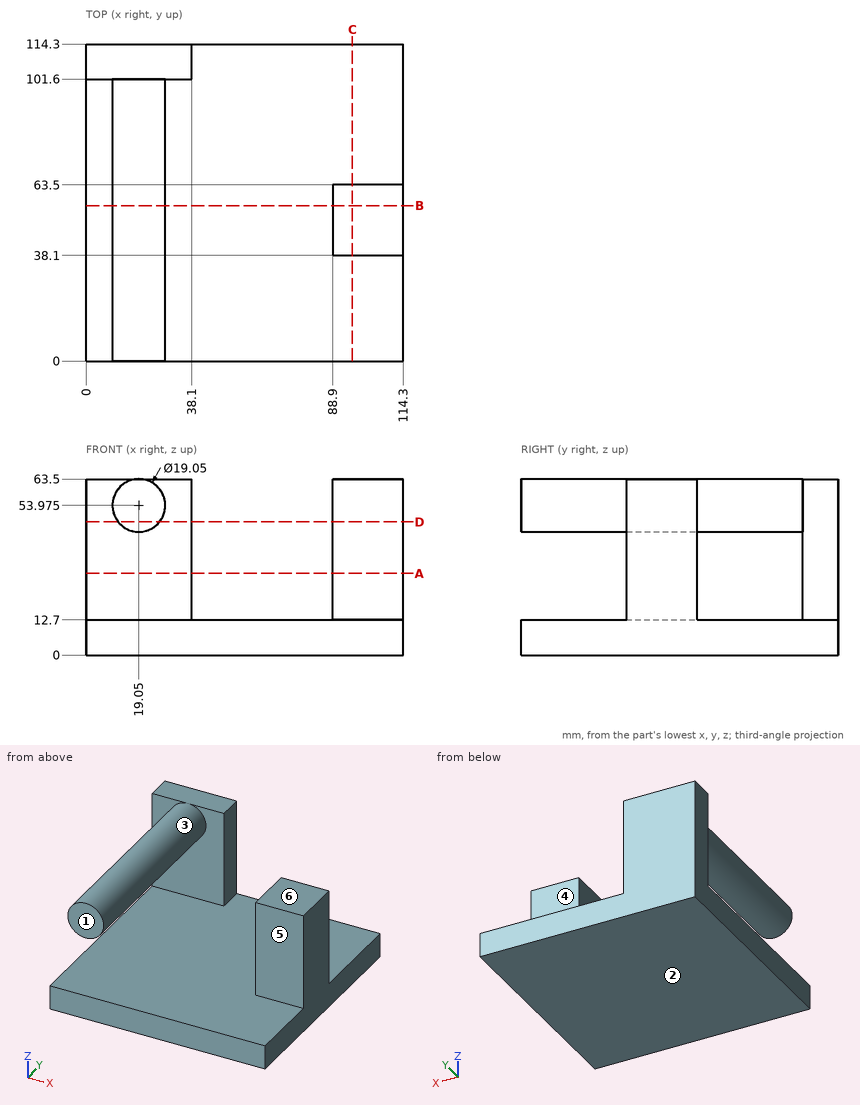
Design review of the part shown in the three views and the two pictorial views. Dimensions are in mm from the part's minimum x, y and z. A direction names the side the tool comes from. Round coordinates to 2 decimals unless told otherwise and drop trailing zeros. Order: outer loops, then holes, each group sorted by start corner. A loop starts at its lowest first (then second) coordinate and runs counter-clockwise, first axis right, second up.
Q1. We need section C-C, the plane x = 96. Give the boundary of the cut face in (y, z), plus the area to 3 significant figures.
Findings below:
outline: (0, 0) - (114.3, 0) - (114.3, 12.7) - (63.5, 12.7) - (63.5, 63.5) - (38.1, 63.5) - (38.1, 12.7) - (0, 12.7) - close
area: 2,740 mm2
Q2. Wall thickness on line 1 (Z direction, x = 62.5, y = 71); line 2 (Y direction, x = 37, z = 52.5); line 3 (X direction, y = 62, z = 27): over which ranges is each line inside the solid? List them lowest first.
Findings below:
line 1: z = 0 to 12.7
line 2: y = 101.6 to 114.3
line 3: x = 88.9 to 114.3
Q3. We need section A-A, the plane z = 29.5. Give the boundary of the cut face in (x, y), plus the area to 3 significant figures.
Findings below:
outline: (0, 101.6) - (38.1, 101.6) - (38.1, 114.3) - (0, 114.3) - close; (88.9, 38.1) - (114.3, 38.1) - (114.3, 63.5) - (88.9, 63.5) - close
area: 1,130 mm2
Q4. We need section D-D, the plane z = 48. Give the boundary of the cut face in (x, y).
Findings below:
outline: (0, 101.6) - (11.63, 101.6) - (11.63, 0) - (26.47, 0) - (26.47, 101.6) - (38.1, 101.6) - (38.1, 114.3) - (0, 114.3) - close; (88.9, 38.1) - (114.3, 38.1) - (114.3, 63.5) - (88.9, 63.5) - close
Q5. Mouldability with a two-part tool opening along Z and no side actions: class the marked faces 1, 2 and 3 as pulls with the +Z half, pulls with the -Z half, needs draft (parallel to the pull), parting line crosses it, or undercut.
Findings below:
face 1: needs draft
face 2: pulls with the -Z half
face 3: undercut
Q6. We need section B-B, the plane y = 56. Give the boundary of the cut face in (x, z) (3 decimals).
Findings below:
outline: (0, 0) - (114.3, 0) - (114.3, 63.5) - (88.9, 63.5) - (88.9, 12.7) - (0, 12.7) - close; circle Ø19.05 at (19.05, 53.975)
Q7. Insertion check: P1, Ø10, axis at y = 106.5, z = 27.5, coming from the +X side; P2, Ø12, axis at y = 67.5, z = 18.5, coming from the -X side; P3, Ø2, axis at x = 96.5, z = 30, coming from the -Y side; P4, Ø20.5, axis at x = 105, z = 27.5, coming from the +Y side. Each pin has a flat end and moves straight along its axis. Give the tip position at first contact, or say it passes through.
Findings below:
P1: stops at x = 38.1
P2: stops at x = 0
P3: stops at y = 38.1
P4: stops at y = 63.5
Q8. Machinability: for the marked faces 4, 5 and 6, which of the approach directions +Z, -Z, +X, -X, +Y, -Y give a long, thin tool a straight path to every point of the face, cutting with its end or side? Answer none if there is none.
Findings below:
face 4: +Z, +X, +Y
face 5: +Z, +X, -Y
face 6: +Z, +X, -X, +Y, -Y
